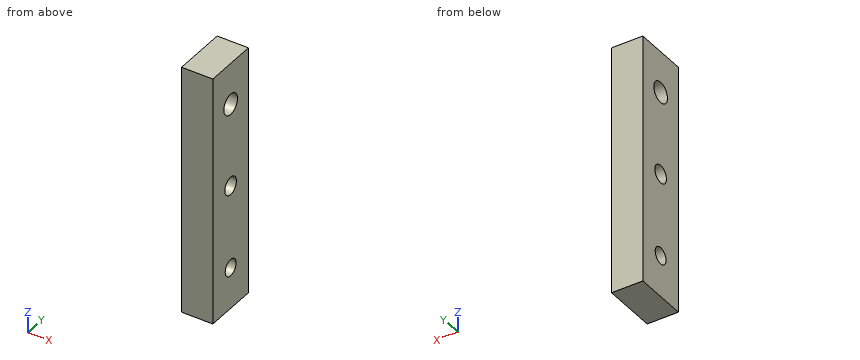
from build123d import *

# Parameters (mm, degrees)
F0_W     = 16.51
F0_H     = 76.2
F0_R     = 2.52436
F0_R_2   = 2.690087
F0_R_3   = 3.157328
F1_DEPTH = 9.525


with BuildPart() as f1:
    # F0 (on Right) → F1 (new body)
    with BuildSketch(Plane.YZ):
        with Locations((-8.255, 38.1)):
            Rectangle(F0_W, F0_H)
        with Locations((-8.255, 12.7)):
            Circle(F0_R, mode=Mode.SUBTRACT)
        with Locations((-8.255, 38.1)):
            Circle(F0_R_2, mode=Mode.SUBTRACT)
        with Locations((-8.255, 63.5)):
            Circle(F0_R_3, mode=Mode.SUBTRACT)
    extrude(amount=F1_DEPTH)


solid = f1.part
Design review of the part built by this model. Coordinates are the model's own, in mm. Give positions to 0.01 mm unless a question says otherwise; leave off trailing zeros. Write each loop counter-clockwise with the first axis right and the second up, starting at its lowest first coordinate (ties: lowest second). Pieces come first, ordered by that corner, then holes. Notation, with made-up numbers: M 80,18 L 98,18 A13 ccw 98,41 Z; hole C 14.25,85 d2. An arc over 180 degrees is marked long. Return JSON: item names as keys, results as strings. Group by question number.
Item 1: Take a section at A-A (z = 63.5). Give the boundary of the cut face in (x, y) (3 decimals), plus the area to 3 significant figures.
Item 2: Take a section at B-B (x = 8.5). Give the boundary of the cut face in (y, z) (3 decimals).
Item 3: Wall thickness on line 1 along Z through (x, y) = (8.25, -9); line 2 along Z through (x, y) = (6.5, -8.5); line 3 along Y through (x, z) = (6.25, 65): over which ranges is each line inside the solid? List them lowest first.
Item 4: Take a section at D-D (z = 12.7). Give the boundary of the cut face in (x, y) (3 decimals), plus the area to 3 significant figures.
Item 5: Take a section at C-C (y = -9.75). Give the boundary of the cut face in (x, z) (3 decimals).
Item 6: Clearance check with a flat-ended pin moving along its axis: pin 1 Ø3 at (y, z) = (-8.255, 12.7) entering from -X. State where the tip first meets the part, or that it passes through.
Return value:
{
 "1": {"outline": "M 0,-16.51 L 9.525,-16.51 L 9.525,-11.412 L 0,-11.412 Z; M 0,-5.098 L 9.525,-5.098 L 9.525,0 L 0,0 Z", "area": "97.1 mm2"},
 "2": {"outline": "M -16.51,0 L 0,0 L 0,76.2 L -16.51,76.2 Z; hole C -8.255,63.5 d6.315; hole C -8.255,38.1 d5.38; hole C -8.255,12.7 d5.049"},
 "3": {"line 1": "z = 0 to 10.29, 15.11 to 35.52, 40.68 to 60.43, 66.57 to 76.2", "line 2": "z = 0 to 10.19, 15.21 to 35.42, 40.78 to 60.35, 66.65 to 76.2", "line 3": "y = -16.51 to -11.03, -5.48 to 0"},
 "4": {"outline": "M 0,-16.51 L 9.525,-16.51 L 9.525,-10.779 L 0,-10.779 Z; M 0,-5.731 L 9.525,-5.731 L 9.525,0 L 0,0 Z", "area": "109 mm2"},
 "5": {"outline": "M 0,0 L 9.525,0 L 9.525,10.666 L 0,10.666 Z; M 0,14.734 L 9.525,14.734 L 9.525,35.864 L 0,35.864 Z; M 0,40.336 L 9.525,40.336 L 9.525,60.719 L 0,60.719 Z; M 0,66.281 L 9.525,66.281 L 9.525,76.2 L 0,76.2 Z"},
 "6": {"pin 1": "passes through"}
}
